```python
from build123d import *

# Parameters (mm, degrees)
SKETCH1_W           = 54
SKETCH1_H           = 10
BOSS_EXTRUDE1_DEPTH = 5
SKETCH3_R           = 1.5
SKETCH3_R_2         = 2
CUT_EXTRUDE1_DEPTH  = 7
FILLET1_R           = 2
SKETCH4_R           = 2.9
SKETCH4_R_2         = 1.5
BOSS_EXTRUDE2_DEPTH = 2.5
CHAMFER1_SIZE       = 1


with BuildPart() as part:
    # Sketch1 → Boss-Extrude1 (new body)
    with BuildSketch(Plane(origin=(0, 0, 0), x_dir=(1, 0, 0), z_dir=(0, 1, 0))):
        Rectangle(SKETCH1_W, SKETCH1_H)
    extrude(amount=BOSS_EXTRUDE1_DEPTH)

    # Sketch3 → Cut-Extrude1 (cut)
    with BuildSketch(Plane(origin=(0, 5, 0), x_dir=(1, 0, 0), z_dir=(0, 1, 0))):
        with Locations(Location((-24.05, 0, 0), (0, 0, 270))):
            Circle(SKETCH3_R)
        with Locations(Location((4, 0, 0), (0, 0, 270))):
            Circle(SKETCH3_R_2)
        with Locations(Location((-8.05, 0, 0), (0, 0, 270))):
            Circle(SKETCH3_R)
        with Locations(Location((20.95, 0, 0), (0, 0, 270))):
            Circle(SKETCH3_R)
    extrude(amount=-CUT_EXTRUDE1_DEPTH, mode=Mode.SUBTRACT)

    # Fillet1
    fillet1_edges = [part.edges().sort_by_distance(p)[0] for p in [
        (27, 2.5, 5),
        (-27, 2.5, 5),
        (-27, 2.5, -5),
        (27, 2.5, -5),
    ]]
    fillet(fillet1_edges, radius=FILLET1_R)

    # Sketch4 → Boss-Extrude2 (add)
    with BuildSketch(Plane.XZ):
        with Locations(Location((-24.05, 0, 0), (0, 0, 270))):
            Circle(SKETCH4_R)
        with Locations(Location((-24.05, 0, 0), (0, 0, 90))):
            Circle(SKETCH4_R_2, mode=Mode.SUBTRACT)
    extrude(amount=BOSS_EXTRUDE2_DEPTH)

    # Chamfer1
    # the kernel refuses this chamfer: 1 mm, written as the material it takes off along each edge
    with BuildSketch(Plane(origin=(-25, 0, -5), x_dir=(0, 0.9996219169112968, -0.027495876610586494), z_dir=(1, 0, 0)), Plane(origin=(25, 5, 5), x_dir=(0, 0.027495876610586487, -0.9996219169112968), z_dir=(-1, 0, 0))) as chamfer1_piece_1:
        Polygon((CHAMFER1_SIZE * 0.999621916911, CHAMFER1_SIZE * 0.0274958766106), (-CHAMFER1_SIZE * 0.0274958766106, CHAMFER1_SIZE * 0.999621916911), (0, 0), align=None)
    extrude(amount=50, mode=Mode.SUBTRACT)
    with BuildSketch(Plane(origin=(-25, 5, -5), x_dir=(0, -0.9996219169112968, -0.027495876610586487), z_dir=(1, 0, 0)), Plane(origin=(25, 0, 5), x_dir=(0, -0.027495876610586365, -0.9996219169112968), z_dir=(-1, 0, 0))) as chamfer1_piece_2:
        Polygon((CHAMFER1_SIZE * 0.999621916911, -CHAMFER1_SIZE * 0.0274958766106), (-CHAMFER1_SIZE * 0.0274958766106, -CHAMFER1_SIZE * 0.999621916911), (0, 0), align=None)
    extrude(amount=50, mode=Mode.SUBTRACT)
    with BuildSketch(Plane(origin=(27, 0, -3), x_dir=(-0.9996219169112968, -0.02749587661058639, 0), z_dir=(0, 0, 1))) as chamfer1_piece_3:
        Polygon((CHAMFER1_SIZE * 0.999621916911, -CHAMFER1_SIZE * 0.0274958766106), (-CHAMFER1_SIZE * 0.0274958766106, -CHAMFER1_SIZE * 0.999621916911), (0, 0), align=None)
    extrude(amount=6, mode=Mode.SUBTRACT)
    with BuildSketch(Plane(origin=(-27, 0, 3), x_dir=(0.9996219169112968, -0.02749587661058639, 0), z_dir=(0, 0, -1))) as chamfer1_piece_4_section:
        Polygon((CHAMFER1_SIZE * 0.999621916911, -CHAMFER1_SIZE * 0.0274958766106), (-CHAMFER1_SIZE * 0.0274958766106, -CHAMFER1_SIZE * 0.999621916911), (0, 0), align=None)
    chamfer1_piece_4 = extrude(amount=6, mode=Mode.PRIVATE)
    chamfer1_piece_4 = chamfer1_piece_4 - Plane(origin=(-24.05, 0.490897833, 0), x_dir=(0, 0, -1), z_dir=(0, 1, 0)) * Cylinder(2.9, 16, mode=Mode.PRIVATE)
    add(chamfer1_piece_4, mode=Mode.SUBTRACT)
    with BuildSketch(Plane(origin=(-25, 0, 3), x_dir=(-1, 0, 0), z_dir=(0, 0, -1))) as chamfer1_piece_5:
        Polygon((2 - CHAMFER1_SIZE, 0), (2, CHAMFER1_SIZE), (2, 0), align=None)
    revolve(axis=Axis((-25, 0, 3), (0, 1, 0)), revolution_arc=90, mode=Mode.SUBTRACT)
    with BuildSketch(Plane(origin=(25, 0, 3), x_dir=(1, 0, 0), z_dir=(0, 0, -1))) as chamfer1_piece_6:
        Polygon((2 - CHAMFER1_SIZE, 0), (2, -CHAMFER1_SIZE), (2, 0), align=None)
    revolve(axis=Axis((25, 0, 3), (0, -1, 0)), revolution_arc=90, mode=Mode.SUBTRACT)
    with BuildSketch(Plane(origin=(-25, 0, -3), x_dir=(0, 0, -1), z_dir=(1, 0, 0))) as chamfer1_piece_7:
        Polygon((2 - CHAMFER1_SIZE, 0), (2, CHAMFER1_SIZE), (2, 0), align=None)
    revolve(axis=Axis((-25, 0, -3), (0, 1, 0)), revolution_arc=90, mode=Mode.SUBTRACT)
    with BuildSketch(Plane(origin=(25, 0, -3), x_dir=(0, 0, -1), z_dir=(-1, 0, 0))) as chamfer1_piece_8:
        Polygon((2 - CHAMFER1_SIZE, 0), (2, -CHAMFER1_SIZE), (2, 0), align=None)
    revolve(axis=Axis((25, 0, -3), (0, -1, 0)), revolution_arc=90, mode=Mode.SUBTRACT)
    with BuildSketch(Plane(origin=(27, 5, -3), x_dir=(-0.9996219169112968, 0.02749587661058651, 0), z_dir=(0, 0, 1)), Plane(origin=(-27, 5, 3), x_dir=(0.9996219169112968, 0.02749587661058651, 0), z_dir=(0, 0, -1))) as chamfer1_piece_9:
        Polygon((CHAMFER1_SIZE * 0.999621916911, CHAMFER1_SIZE * 0.0274958766106), (-CHAMFER1_SIZE * 0.0274958766106, CHAMFER1_SIZE * 0.999621916911), (0, 0), align=None)
    extrude(amount=6, mode=Mode.SUBTRACT)
    with BuildSketch(Plane(origin=(-25, 5, 3), x_dir=(-1, 0, 0), z_dir=(0, 0, -1))) as chamfer1_piece_10:
        Polygon((2 - CHAMFER1_SIZE, 0), (2, -CHAMFER1_SIZE), (2, 0), align=None)
    revolve(axis=Axis((-25, 5, 3), (0, 1, 0)), revolution_arc=90, mode=Mode.SUBTRACT)
    with BuildSketch(Plane(origin=(25, 5, 3), x_dir=(1, 0, 0), z_dir=(0, 0, -1))) as chamfer1_piece_11:
        Polygon((2 - CHAMFER1_SIZE, 0), (2, CHAMFER1_SIZE), (2, 0), align=None)
    revolve(axis=Axis((25, 5, 3), (0, -1, 0)), revolution_arc=90, mode=Mode.SUBTRACT)
    with BuildSketch(Plane(origin=(-25, 5, -3), x_dir=(0, 0, -1), z_dir=(1, 0, 0))) as chamfer1_piece_12:
        Polygon((2, -CHAMFER1_SIZE), (2 - CHAMFER1_SIZE, 0), (2, 0), align=None)
    revolve(axis=Axis((-25, 5, -3), (0, 1, 0)), revolution_arc=90, mode=Mode.SUBTRACT)
    with BuildSketch(Plane(origin=(25, 5, -3), x_dir=(0, 0, -1), z_dir=(-1, 0, 0))) as chamfer1_piece_13:
        Polygon((2, CHAMFER1_SIZE), (2 - CHAMFER1_SIZE, 0), (2, 0), align=None)
    revolve(axis=Axis((25, 5, -3), (0, -1, 0)), revolution_arc=90, mode=Mode.SUBTRACT)


solid = part.part
```
The listing builds one solid part. Answer for the finished solid, in the listing's coordinates (mm). A direction names the side the tool comes from. Round coordinates to 2 decimals unless told otherwise and drop trailing zeros. Order: outer loops, then holes, each group sorted by start corner. A loop starts at its lowest first (then second) coordinate and runs counter-clockwise, first axis right, second up. Notation, with made-up numbers: (11.5, 70.5) - (61.5, 70.5) arc R32 ccw to (61.5, 103.5) - close; hole circle Ø2 at (74.25, -21). An arc over 180 degrees is marked (long way). Put each result on its own line as item: value. Start each with the question number.
(1) Determine the mould class of faces 3 (the flat face through (-0.4, 0.5, -4.5)), 4 (the cylindrical face through (22.437, 2.535, -0.195)), 5 (the flat face through (-26.5, 4.5, 0)) for opening direction Z: released by +Z, released by -Z, zero draft, split by the parting line, or undercut.
(2) Find section D-D (x = 20.95). Give the vertices of the cut face in (y, z).
(3) For faces 1 (the flat face through (-26.8, 0.8, 1.4)), 2 (the conical face through (-26, 4.6, 3.98)), determine the directions among +Z, -Z, +X, -X, +Y, -Y from which every point of the face is accessible in a straight line to the end or side of a thin tool.
(4) Find section C-C (z = -0.75). Give the vertices of the cut face in (x, y).
(5) Straight lines are drawn through the part: probe 1 along X at (y, z) = (3.4, 0); probe 2 along Z at (x, y) = (-24.05, 2); probe 3 along Y at (x, z) = (23.5, -3.75). For each, find the intervals that lie inside material, in ascending order. Write a range as from..to.
(6) Find section A-A (x = 4). Give the vertices of the cut face in (y, z), plus the area to 3 significant figures.
(7) Find section B-B (y = 2.5). Give the vertices of the cut face in (x, z).
(8) Given P1, Ø4, axis at x = 3, z = 2, coming from the -Y side, flat-ended and moving along its own axis, determine where the tip first touches the part or whether it passes through.
Reply:
1. face 3: released by -Z
1. face 4: undercut
1. face 5: zero draft
2. outline: (0, -4) - (1, -5) - (4, -5) - (5, -4) - (5, -1.5) - (0, -1.5) - close; (0, 1.5) - (5, 1.5) - (5, 4) - (4, 5) - (1, 5) - (0, 4) - close
3. face 1: -X, -Y
3. face 2: +Z, -X, +Y
4. outline: (-27, 1) - (-26.85, 0.85) - (-26.85, -2.5) - (-25.35, -2.5) - (-25.35, 5) - (-26, 5) - (-27, 4) - close; (-22.75, -2.5) - (-21.25, -2.5) - (-21.25, 0) - (-9.35, 0) - (-9.35, 5) - (-22.75, 5) - close; (-6.75, 0) - (2.15, 0) - (2.15, 5) - (-6.75, 5) - close; (5.85, 0) - (19.65, 0) - (19.65, 5) - (5.85, 5) - close; (22.25, 0) - (26, 0) - (27, 1) - (27, 4) - (26, 5) - (22.25, 5) - close
5. probe 1: -27..-25.55, -22.55..-9.55, -6.55..2, 6..19.45, 22.45..27
5. probe 2: -5..-1.5, 1.5..5
5. probe 3: 0..5
6. outline: (0, -4) - (1, -5) - (4, -5) - (5, -4) - (5, -2) - (0, -2) - close; (0, 2) - (5, 2) - (5, 4) - (4, 5) - (1, 5) - (0, 4) - close
6. area: 28.0 mm^2
7. outline: (-27, -3) arc R2 ccw to (-25, -5) - (25, -5) arc R2 ccw to (27, -3) - (27, 3) arc R2 ccw to (25, 5) - (-25, 5) arc R2 ccw to (-27, 3) - close; hole circle Ø3 at (-24.05, 0); hole circle Ø3 at (-8.05, 0); hole circle Ø4 at (4, 0); hole circle Ø3 at (20.95, 0)
8. P1: y = 0
